Autodesk Fusion 360 part; units mm, degrees
sketch "Sketch1" plane through (0, 0, 0) normal (0, 0, 1) x (1, 0, 0)
  circle A0 centre (0, 0) radius 22
  dimension "d1" = 44
extrude "Extrude1" add sketch "Sketch1" along normal blind 30
sketch "Sketch2" plane through (0, 0, 30) normal (0, 0, 1) x (-1, 0, 0)
  circle A0 centre (0, 0) radius 22
  circle A1 centre (0, 0) radius 20.3
  dimension "d4" = 40.6
extrude "Extrude2" cut sketch "Sketch2" against normal blind 28 contours A1
ref_plane "WorkPlane1" through (22, 0, 0) normal (1, 0, 0) x (0, 1, 0)
sketch "Sketch6" plane through (22, 0, 0) normal (1, 0, 0) x (0, 1, 0)
  line L0 (-3, 6) -> (3, 6)
  line L1 (3, 6) -> (3, 0)
  line L2 (3, 0) -> (-3, 0)
  line L3 (-3, 0) -> (-3, 6)
  line L4 (-3, 6) -> (3, 0) construction
  line L5 (3, 6) -> (-3, 0) construction
  point P0 (0, 3)
  dimension "d15" = 6
  dimension "d16" = 6
extrude "Extrude5" add sketch "Sketch6" along normal blind 4 and the other way up to surface second end surface at (21.8907, -2.1905, 20)
sketch "Sketch7" plane through (0, 0, 0) normal (0, 0, -1) x (1, 0, 0)
  line L0 (21.7945, -3) -> (26, -3)
  line L1 (26, -3) -> (26, 3)
  line L2 (26, 3) -> (21.7945, 3)
  line L3 (25.5, -2.5) -> (22.5, -2.5)
  line L4 (22.5, -2.5) -> (22.5, 2.5)
  line L5 (22.5, 2.5) -> (25.5, 2.5)
  line L6 (25.5, 2.5) -> (25.5, -2.5)
  line L7 (25.5, -2.5) -> (22.5, 2.5) construction
  line L8 (22.5, -2.5) -> (25.5, 2.5) construction
  arc A0 (21.7945, 3) -> (21.7945, -3) centre (0, 0) ccw
  point P0 (24, 0)
  dimension "d19" = 3
  dimension "d20" = 5
extrude "Extrude6" cut sketch "Sketch7" against normal blind 3 contours L3 L4 L5 L6
sketch "Sketch8" plane through (0, 0, 0) normal (0, 0, -1) x (1, 0, 0)
  line L0 (22.5, -2.5) -> (22.5, 2.5)
  line L1 (22.5, 2.5) -> (25.5, 2.5)
  line L2 (25.5, 2.5) -> (25.5, -2.5)
  line L3 (25.5, -2.5) -> (22.5, -2.5)
  arc A0 (21.7945, 3) -> (21.7945, -3) centre (0, 0) ccw
  line L4 (21.7945, -3) -> (26, -3)
  line L5 (26, -3) -> (26, 3)
  line L6 (26, 3) -> (21.7945, 3)
  circle A1 centre (0, 0) radius 8.5
  circle A2 centre (0, 0) radius 7.2
  dimension "d25" = 17
  dimension "d26" = 14.4
extrude "Extrude7" add sketch "Sketch8" along normal blind 4.5 contours A1
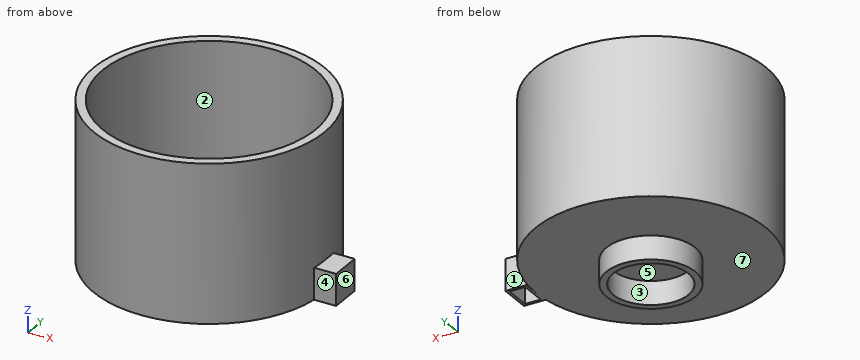
Could you check a few things on this model? Use its own coordinates, in mm. Face numbers are marked on the shaded views. A direction names the side the tool comes from. Give positions to 0.01 mm unless a question says otherwise; leave off trailing zeros. Order: outer loops, then holes, each group sorted by start corner. A loop starts at its lowest first (then second) coordinate and runs counter-clockwise, first axis right, second up. Notation, with made-up numbers: (4, -29.5) -> (36, -29.5) arc R20 cw to (36, 3.5) -> close; hole circle Ø7 at (83, 33). An arc over 180 degrees is marked (long way). Answer in a Markdown table with one row per item. Add a question column.
Item 1: Imagine slicing it at D-D (y = 5). List the corners of the cut face in (x, z) for me.
Item 2: Imagine slicing it at C-C (z = 27.5). List the corners of the cut face in (x, y) for me, and give its area (3 significant figures).
Item 3: Imagine slicing it at B-B (y = 18). List the corners of the cut face in (x, z) for me.
Item 4: For the marked faces 1, 2, 3 and 4, which set-ups out of +Z, -Z, +X, -X, +Y, -Y let a thin tool reach every point of the face, with its end or its side?
Item 5: Please list where these lines run through material, in increasing order: probe 1 along X at (y, z) = (0, -1.65); probe 2 along Y at (x, z) = (-0.5, 23.5).
Item 6: Imagine slicing it at A-A (x = 0). List the corners of the cut face in (y, z) for me.
Item 7: I'm going to push flat-ended pins straight in: P1, Ø2.5, axis at x = 23.5, z = 2, coming from the -Y side; P2, Ø10, axis at x = -9.5, y = 11, coming from the +Z side; P3, Ø4, axis at y = 13, z = 1, coming from the -X side. Where does each tip first touch, or does it pass through?
Item 8: We'd pull the mould along X, two halves only. Please class the marked faces 5, 6 and 7: pulls with the +X half, pulls with the -X half, needs draft (parallel to the pull), parting line crosses it, or undercut.
Result:
| question | item | result |
|---|---|---|
| 1 | outline | (-21.42, 0) -> (-6.87, 0) -> (-6.87, -4.5) -> (-5.18, -4.5) -> (-5.18, 0) -> (5.18, 0) -> (5.18, -4.5) -> (6.87, -4.5) -> (6.87, 0) -> (21.42, 0) -> (21.42, 30) -> (19.67, 30) -> (19.67, 2) -> (-19.67, 2) -> (-19.67, 30) -> (-21.42, 30) -> close |
| 2 | outline | circle Ø44 at (0, 0); hole circle Ø40.6 at (0, 0) |
| 2 | area | 226 mm2 |
| 3 | outline | (-12.65, 0) -> (12.65, 0) -> (12.65, 30) -> (9.39, 30) -> (9.39, 2) -> (-9.39, 2) -> (-9.39, 30) -> (-12.65, 30) -> close |
| 4 | face 1 | +Z, -Z, +X, +Y |
| 4 | face 2 | +Z |
| 4 | face 3 | -Z |
| 4 | face 4 | +Z, -Z, +X, -Y |
| 5 | probe 1 | -8.5 to -7.2, 7.2 to 8.5 |
| 5 | probe 2 | -21.99 to -20.29, 20.29 to 21.99 |
| 6 | outline | (-22, 0) -> (-8.5, 0) -> (-8.5, -4.5) -> (-7.2, -4.5) -> (-7.2, 0) -> (7.2, 0) -> (7.2, -4.5) -> (8.5, -4.5) -> (8.5, 0) -> (22, 0) -> (22, 30) -> (20.3, 30) -> (20.3, 2) -> (-20.3, 2) -> (-20.3, 30) -> (-22, 30) -> close |
| 7 | P1 | y = -3 |
| 7 | P2 | z = 2 |
| 7 | P3 | x = -19.05 |
| 8 | face 5 | undercut |
| 8 | face 6 | pulls with the +X half |
| 8 | face 7 | needs draft |
